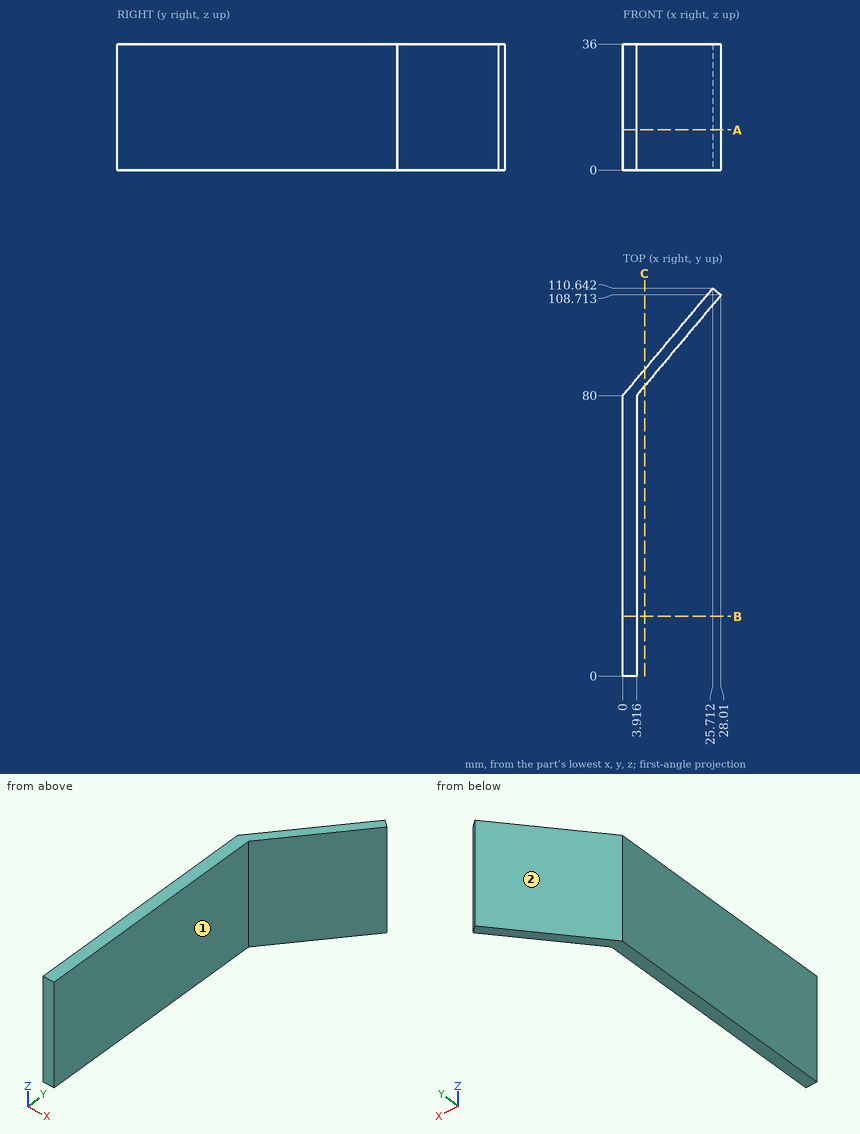
Job drawing, mm, ordinate dimensions from the low corner. One solid piece. A direction names the side the tool comes from. Give positions to 0.01 mm unless a question says otherwise; leave off trailing zeros. Loops run counter-clockwise (first coordinate to the right, second up) from the corner with the lowest first, then second, coordinate; pieces in that order, holes last. Notation, with made-up numbers: (63, 5.5) - (117, 5.5) arc R34 ccw to (117, 39.5) - close; hole circle Ø5 at (11, 46). An arc over 180 degrees is marked (long way). Use one line per item in the form item = value.
(1) Drill centre lines: L1, parallel to X at y = 38, z = 16.5; L2, parallel to Y at x = 9.5, z = 30 (1 decimal); L3, parallel to Y at x = 24.25, z = 30 (1 decimal). Where is each one in solid material? Low to high.
Determined:
L1 = 0 to 3.92
L2 = 86.7 to 91.3
L3 = 104.2 to 108.9
(2) 3-axis set-ups, long thin cutter, end or side, ignore diameter. For the marked faces 1 and 2: which of +Z, -Z, +X, -X, +Y, -Y reach the whole face in a straight line?
Determined:
face_1 = +Z, -Z, +X, -Y
face_2 = +Z, -Z, -X, +Y
(3) Cut at B-B (y = 17). Give the cut face in (x, z).
Determined:
outline = (0, 0) - (3.92, 0) - (3.92, 36) - (0, 36) - close
(4) Drop flat-ended pins along their axis: P1, Ø1.5, axis at x = 9, z = 9, coming from the +Y side; P2, Ø6, axis at y = 86.5, z = 8, coming from the -X side; P3, Ø10, axis at y = 31.5, z = 30.5, coming from the -X side; P4, Ø11, axis at y = 31, z = 15.5, coming from the +X side. Give the stop position or say it passes through.
Determined:
P1 = 91.62
P2 = 2.94
P3 = 0
P4 = 3.92
(5) Cut at C-C (x = 6.25). Give the cut face in (y, z), then the cut area to 3 significant figures.
Determined:
outline = (82.78, 0) - (87.45, 0) - (87.45, 36) - (82.78, 36) - close
area = 168 mm^2
(6) Cut at A-A (z = 11.5). Give the cut face in (x, y).
Determined:
outline = (0, 0) - (3.92, 0) - (3.92, 80) - (28.01, 108.71) - (25.71, 110.64) - (0, 80) - close
